Read the model definition and answer for the solid it produces. Units are mm, in the model's axes. A direction names the side the tool comes from. Round coordinates to 2 decimals unless told otherwise and drop trailing zeros. Write each loop counter-clockwise with the first axis right and the second up, starting at its lowest first coordinate (ties: lowest second). Pieces come first, ordered by that corner, then holes. Notation, with made-up numbers: (5, -19.75) -> (12, -19.75) arc R31 ccw to (12, 10.25) -> close; hole circle Ø1 at (5, -16.5). An arc over 180 degrees is marked (long way). Return JSON: item names as keys, results as strings. Group by question number.
(1) A cutting plane is placed at A-A on z = -22. Give the vertices of the cut face in (x, y) (3 decimals), then the cut area to 3 significant figures.
(2) Straight lines are drawn through the part: line 1 (Y direction, x = 2.6, z = -17) (3 decimals); line 2 (Y direction, x = 1.5, z = -31) (3 decimals); line 3 (Z direction, x = 0.35, y = 10.5). For each, find the intervals that lie inside material, in ascending order.
(3) Given pin 1 (1 mm diameter, centred on x = 2, y = 1.5, fed in from +Z); pin 2 (1 mm diameter, centred on x = 2, z = -66.5, fed in from -Y) (3 decimals); pin 3 (1.6 mm diameter, centred on x = 1.5, y = 30.5, fed in from +Z), each flat-ended and moving along its own axis, determine where each tip first touches the part or whether it passes through.
(4) A cutting plane is placed at B-B on y = 22.5. State how many separate pieces and enclosed holes the cut face has, then the cut area to 3 significant figures.
(5) A cutting plane is placed at C-C on y = 43.5. Give the vertices of the cut face in (x, z) (3 decimals).
(6) The mould has two halves that part along Y. Classify faces 1 (the flat face through (1.57, 27.06, -76.47)), 2 (the flat face through (0, 25, -50)), 3 (the flat face through (2, 20.675, -21)): released by +Y, released by -Y, zero draft, split by the parting line, or undercut.
(7) A cutting plane is placed at D-D on y = 52.5. Give the vertices of the cut face in (x, z) (3 decimals).
(8) For faces 4 (the flat face through (2, 29, -15.325)), 5 (the flat face through (1.6, 51.6, -85.4)), 6 (the flat face through (2, 45.958, -42)), determine the directions among +Z, -Z, +X, -X, +Y, -Y from which every point of the face is accessible in a straight line to the end or side of a thin tool.
```python
from build123d import *

# Parameters (mm, degrees)
BOSS_EXTRUDE1_DEPTH = 3.175
SKETCH2_W           = 27.85
SKETCH2_H           = 35.791497658
CUT_EXTRUDE1_DEPTH  = 4.1750001
SKETCH3_W           = 10.508
SKETCH3_H           = 3.175
BOSS_EXTRUDE2_DEPTH = 3.175
SKETCH4_W           = 22.5
SKETCH4_H           = 3.175
CUT_EXTRUDE2_DEPTH  = 4.1750001
SKETCH5_W           = 39.932212354
SKETCH5_H           = 4.644211625
CUT_EXTRUDE3_DEPTH  = 10


with BuildPart() as part:
    # Sketch1 → Boss-Extrude1 (new body)
    with BuildSketch(Plane(origin=(0, 0, 0), x_dir=(0, 0, -1), z_dir=(1, 0, 0))):
        with BuildLine():
            Line((0, 0), (70, 0))
            Line((70, 0), (90.5212086, 56.381557247))
            add(Edge.make_bspline(
                [(-11.490666647, 9.641814145), (19.4560829, 46.522714097), (48.01605029, 71.852169675), (90.5212086, 56.381557247)],
                knots=[0, 0, 0, 0, 1, 1, 1, 1], degree=3))
            Line((-11.490666647, 9.641814145), (0, 0))
        make_face()
    extrude(amount=BOSS_EXTRUDE1_DEPTH)

    # Sketch2 → Cut-Extrude1 (cut, through all)
    with BuildSketch(Plane.ZY):
        with Locations((-29.25, 38.570748829)):
            Rectangle(SKETCH2_W, SKETCH2_H)
    extrude(amount=-CUT_EXTRUDE1_DEPTH, mode=Mode.SUBTRACT)

    # Sketch3 → Boss-Extrude2 (add)
    with BuildSketch(Plane.ZY):
        Polygon((-43.175, 56.466497658), (-43.175, 45.958497658), (-40.79375, 45.958497658), align=None)
        with Locations((-31.35, 22.2625)):
            Rectangle(SKETCH3_W, SKETCH3_H)
    extrude(amount=-BOSS_EXTRUDE2_DEPTH)

    # Sketch4 → Cut-Extrude2 (cut, through all)
    with BuildSketch(Plane.ZY):
        Polygon((-83.262432737, 45.721313442), (-86.245956808, 44.635399487), (-90.5212086, 56.381557247), (-87.537684529, 57.467471202), align=None)
        Polygon((-79.842231304, 36.324387235), (-73.001828437, 17.530534819), (-75.985352508, 16.444620864), (-82.825755375, 35.238473279), align=None)
        Polygon((-72.565151075, 7.047694656), (-70, 0), (-62.5, 0), (-62.5, 3.175), (-67.776841066, 3.175), (-69.581627004, 8.133608611), align=None)
        with Locations((-36.25, 1.5875)):
            Rectangle(SKETCH4_W, SKETCH4_H)
        Polygon((-10, 3.175), (-10, 0), (0, 0), (5.745333323, 4.820907073), (3.704482663, 7.25309818), (-1.155605494, 3.175), align=None)
    extrude(amount=-CUT_EXTRUDE2_DEPTH, mode=Mode.SUBTRACT)

    # Sketch5 → Cut-Extrude3 (cut)
    with BuildSketch(Plane.ZY):
        with Locations((-35.043485806, 11.047370883)):
            Rectangle(SKETCH5_W, SKETCH5_H)
    extrude(amount=-CUT_EXTRUDE3_DEPTH, mode=Mode.SUBTRACT)


solid = part.part
```
Checks:
{
 "1": {"outline": "(0, 0) -> (3.175, 0) -> (3.175, 8.725) -> (0, 8.725) -> close; (0, 13.369) -> (3.175, 13.369) -> (3.175, 20.675) -> (0, 20.675) -> close", "area": "50.9 mm^2"},
 "2": {"line 1": "y = 0 to 8.725, 13.369 to 20.675", "line 2": "y = 3.175 to 8.725, 13.369 to 23.85", "line 3": "z = -73.82 to -55.01, -15.08 to 10.77"},
 "3": {"pin 1": "stops at z = -10", "pin 2": "stops at y = 3.175", "pin 3": "stops at z = -6.48"},
 "4": {"separate pieces": "3", "enclosed holes": "0", "area": "183 mm^2"},
 "5": {"outline": "(0, -85.833) -> (3.175, -85.833) -> (3.175, -43.175) -> (0, -43.175) -> close"},
 "6": {"face 1": "undercut", "face 2": "zero draft", "face 3": "released by +Y"},
 "7": {"outline": "(0, -85.73) -> (3.175, -85.73) -> (3.175, -42.276) -> (0, -42.276) -> close"},
 "8": {"face 4": "+X, -X, +Y", "face 5": "-Z, +X, -X", "face 6": "+Z, +X, -X"}
}
